The model under review builds one solid part; all positions refer to its coordinate system, in mm. Face numbers are marked on the shaded views. Round coordinates to 2 decimals unless told otherwise and drop trailing zeros. Order: outer loops, then holes, each group sorted by start corner. A loop starts at its lowest first (then second) coordinate and runs counter-clockwise, first axis right, second up. Notation, with made-up numbers: M -25.75,4.5 L -9.75,4.5 A25 cw -9.75,37.5 Z; hole C 7.25,-4.5 d6. An arc over 180 degrees is marked long. One line per item, written item: value. Start each with the question number.
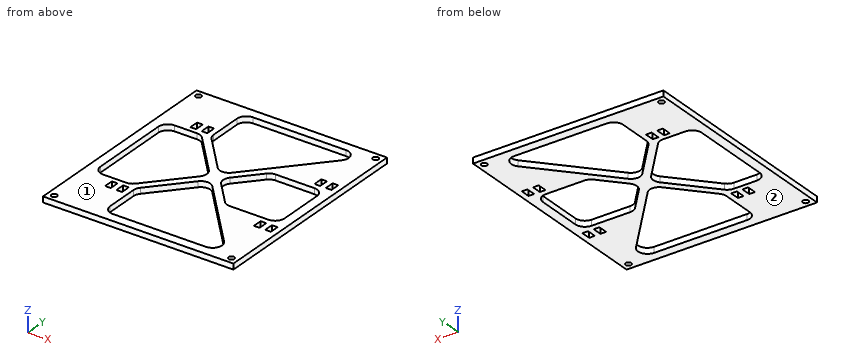
from build123d import *

# Parameters (mm, degrees)
SKETCH1_W           = 101
SKETCH1_H           = 114
SKETCH1_R           = 1.5
BOSS_EXTRUDE1_DEPTH = 3
SKETCH2_W           = 3
SKETCH2_H           = 5
BOSS_EXTRUDE2_DEPTH = 3
SKETCH2_2_W         = 3
SKETCH2_2_H         = 5
CUT_EXTRUDE1_DEPTH  = 3
SKETCH3_W           = 3
SKETCH3_H           = 5
BOSS_EXTRUDE3_DEPTH = 3
SKETCH3_2_W         = 3
SKETCH3_2_H         = 5
CUT_EXTRUDE2_DEPTH  = 3
FILLET4_R           = 5


with BuildPart() as part:
    # Sketch1 → Boss-Extrude1 (new body)
    with BuildSketch(Plane.XY):
        with Locations((21.186424942, -0.122053896)):
            Rectangle(SKETCH1_W, SKETCH1_H)
        with Locations((68.186424942, 53.377946104)):
            Circle(SKETCH1_R, mode=Mode.SUBTRACT)
        with Locations((68.186424942, -53.622053896)):
            Circle(SKETCH1_R, mode=Mode.SUBTRACT)
        with Locations((-25.813575058, -53.622053896)):
            Circle(SKETCH1_R, mode=Mode.SUBTRACT)
        with Locations((-25.813575058, 53.377946104)):
            Circle(SKETCH1_R, mode=Mode.SUBTRACT)
        with BuildLine():
            Line((-11.101826841, -52.122053896), (53.474676725, -52.122053896))
            ThreePointArc((53.474676725, -52.122053896), (58.034200224, -49.174063999), (57.21715204, -43.806352082))
            Line((57.21715204, -43.806352082), (24.928900257, -7.362186703))
            ThreePointArc((24.928900257, -7.362186703), (21.186424942, -5.677888517), (17.443949627, -7.362186703))
            Line((17.443949627, -7.362186703), (-14.844302156, -43.806352082))
            ThreePointArc((-14.844302156, -43.806352082), (-15.66135034, -49.174063999), (-11.101826841, -52.122053896))
        make_face(mode=Mode.SUBTRACT)
        with BuildLine():
            Line((-24.313575058, -35.279090562), (-24.313575058, 35.03498277))
            ThreePointArc((-24.313575058, 35.03498277), (-21.086654783, 39.710043015), (-15.571099743, 38.350684584))
            Line((-15.571099743, 38.350684584), (15.576801163, 3.193647918))
            ThreePointArc((15.576801163, 3.193647918), (16.834325848, -0.122053896), (15.576801163, -3.43775571))
            Line((15.576801163, -3.43775571), (-15.571099743, -38.594792376))
            ThreePointArc((-15.571099743, -38.594792376), (-21.086654783, -39.954150806), (-24.313575058, -35.279090562))
        make_face(mode=Mode.SUBTRACT)
        with BuildLine():
            Line((-11.101826841, 51.877946104), (53.474676725, 51.877946104))
            ThreePointArc((53.474676725, 51.877946104), (58.034200224, 48.929956208), (57.21715204, 43.56224429))
            Line((57.21715204, 43.56224429), (24.928900257, 7.118078911))
            ThreePointArc((24.928900257, 7.118078911), (21.186424942, 5.433780725), (17.443949627, 7.118078911))
            Line((17.443949627, 7.118078911), (-14.844302156, 43.56224429))
            ThreePointArc((-14.844302156, 43.56224429), (-15.66135034, 48.929956208), (-11.101826841, 51.877946104))
        make_face(mode=Mode.SUBTRACT)
        with BuildLine():
            Line((66.686424942, -35.279090562), (66.686424942, 35.03498277))
            ThreePointArc((66.686424942, 35.03498277), (63.459504668, 39.710043015), (57.943949627, 38.350684584))
            Line((57.943949627, 38.350684584), (26.796048721, 3.193647918))
            ThreePointArc((26.796048721, 3.193647918), (25.538524036, -0.122053896), (26.796048721, -3.43775571))
            Line((26.796048721, -3.43775571), (57.943949627, -38.594792376))
            ThreePointArc((57.943949627, -38.594792376), (63.459504668, -39.954150806), (66.686424942, -35.279090562))
        make_face(mode=Mode.SUBTRACT)
    extrude(amount=BOSS_EXTRUDE1_DEPTH)

    # Sketch2 → Boss-Extrude2 (add)
    # profile 1 of 2: a face of its own
    with BuildSketch(Plane.XY.offset(3)):
        Polygon((69.525635116, 16.877946104), (38.919856763, 16.877946104), (69.525635116, 52.236469223), align=None)
        with Locations((67.186424942, 22.377946104)):
            Rectangle(SKETCH2_W, SKETCH2_H, mode=Mode.SUBTRACT)
        with Locations((61.186424942, 22.377946104)):
            Rectangle(SKETCH2_W, SKETCH2_H, mode=Mode.SUBTRACT)
    # profile 2 of 2: a face of its own
    with BuildSketch(Plane.XY.offset(3)):
        Polygon((69.539183497, -17.122053896), (38.919856763, -17.122053896), (69.539183497, -51.682482091), align=None)
        with Locations((67.186424942, -22.622053896)):
            Rectangle(SKETCH2_W, SKETCH2_H, mode=Mode.SUBTRACT)
        with Locations((61.186424942, -22.622053896)):
            Rectangle(SKETCH2_W, SKETCH2_H, mode=Mode.SUBTRACT)
    extrude(amount=-BOSS_EXTRUDE2_DEPTH)

    # Sketch2_2 → Cut-Extrude1 (cut)
    with BuildSketch(Plane.XY.offset(3)):
        with Locations((67.186424942, 22.377946104)):
            Rectangle(SKETCH2_2_W, SKETCH2_2_H)
        with Locations((67.186424942, -22.622053896)):
            Rectangle(SKETCH2_2_W, SKETCH2_2_H)
    extrude(amount=-CUT_EXTRUDE1_DEPTH, mode=Mode.SUBTRACT)

    # Sketch3 → Boss-Extrude3 (add)
    with BuildSketch(Plane.XY.offset(3)):
        Polygon((-0.794496608, -27.948155721), (-0.794496608, -52.122053896), (-24.313575058, -52.122053896), (-24.313575058, -26.468030189), (-0.794496608, -26.468030189), align=None)
        with Locations((-11.294496608, -31.622053896)):
            Rectangle(SKETCH3_W, SKETCH3_H, mode=Mode.SUBTRACT)
        with Locations((-5.294496608, -31.622053896)):
            Rectangle(SKETCH3_W, SKETCH3_H, mode=Mode.SUBTRACT)
    boss_extrude3 = extrude(amount=-BOSS_EXTRUDE3_DEPTH)

    # Sketch3_2 → Cut-Extrude2 (cut)
    with BuildSketch(Plane.XY.offset(3)):
        with Locations((-11.294496608, -31.622053896)):
            Rectangle(SKETCH3_2_W, SKETCH3_2_H)
        with Locations((-5.294496608, -31.622053896)):
            Rectangle(SKETCH3_2_W, SKETCH3_2_H)
    cut_extrude2 = extrude(amount=-CUT_EXTRUDE2_DEPTH, mode=Mode.SUBTRACT)

    # Mirror1: Boss-Extrude3, Cut-Extrude2 across plane
    add(boss_extrude3.mirror(Plane.ZX))
    add(cut_extrude2.mirror(Plane.ZX), mode=Mode.SUBTRACT)

    # Fillet4
    fillet4_edges = [part.edges().sort_by_distance(p)[0] for p in [
        (38.919856763, 16.877946104, 1.5),
        (66.686424942, 16.877946104, 1.5),
        (66.686424942, -17.122053896, 1.5),
        (38.919856763, -17.122053896, 1.5),
        (-0.794496608, -27.948155721, 1.5),
        (-24.313575058, -26.468030189, 1.5),
        (-0.794496608, -52.122053896, 1.5),
        (-4.827213946, -26.468030189, 1.5),
        (-0.794496608, 51.877946104, 1.5),
        (-5.043484884, 26.468030189, 1.5),
        (-24.313575058, 26.468030189, 1.5),
        (-0.794496608, 27.70404793, 1.5),
    ]]
    fillet(fillet4_edges, radius=FILLET4_R)


solid = part.part
Item 1: The part is to be moulded in two halves that separate along Z. For the marked faces 1 and 2, say which applies: pulls with the +Z half, pulls with the -Z half, needs draft (parallel to the pull), parting line crosses it, or undercut.
Item 2: Consider section A-A, the plane x = 44. Give the boundary of the cut face in (y, z).
Item 3: Consider section C-C, the plane x = 19.5. Give the boundary of the cut face in (y, z), then the cut area to 3 significant figures.
Item 4: Clearance check with a flat-ended pin moving along its axis: P1, Ø2.5, axis at x = 68.19, y = -53.62, coming from the +Z side. State where the tip first meets the part, or that it passes through.
Item 5: Consider section D-D, the plane x = 55. Give the boundary of the cut face in (y, z).
Item 6: Consider section B-B, the plane y = 36. Give the boundary of the cut face in (x, z), then the cut area to 3 significant figures.
Item 7: Wall thickness on L1, parallel to Y at x = -12, z = 0.55; L2, parallel to X at y = 4.5, z = 1.6; L3, parallel to Y at x = 42, z = 1.65: over which ranges is each line inside the solid? List them lowest first.
Computed:
1. face 1: pulls with the +Z half
1. face 2: pulls with the -Z half
2. outline: M -57.12,0 L -52.12,0 L -52.12,3 L -57.12,3 Z; M -28.89,0 L -17.12,0 L -17.12,3 L -28.89,3 Z; M 16.88,0 L 28.64,0 L 28.64,3 L 16.88,3 Z; M 51.88,0 L 56.88,0 L 56.88,3 L 51.88,3 Z
3. outline: M -57.12,0 L -52.12,0 L -52.12,3 L -57.12,3 Z; M -5.97,0 L 5.73,0 L 5.73,3 L -5.97,3 Z; M 51.88,0 L 56.88,0 L 56.88,3 L 51.88,3 Z
3. area: 65.1 mm^2
4. P1: passes through
5. outline: M -57.12,0 L -51.88,0 L -51.88,3 L -57.12,3 Z; M -41.3,0 L -17.12,0 L -17.12,3 L -41.3,3 Z; M 16.88,0 L 41.06,0 L 41.06,3 L 16.88,3 Z; M 51.64,0 L 56.88,0 L 56.88,3 L 51.64,3 Z
6. outline: M -29.31,0 L -0.79,0 L -0.79,3 L -29.31,3 Z; M 50.52,0 L 71.69,0 L 71.69,3 L 50.52,3 Z
6. area: 149 mm^2
7. L1: y = -57.12 to -34.12, -29.12 to -26.47, 26.47 to 29.12, 34.12 to 56.88
7. L2: x = -29.31 to -24.31, 14.42 to 27.95, 66.69 to 71.69
7. L3: y = -57.12 to -52.12, -26.63 to -17.12, 16.88 to 26.39, 51.88 to 56.88
